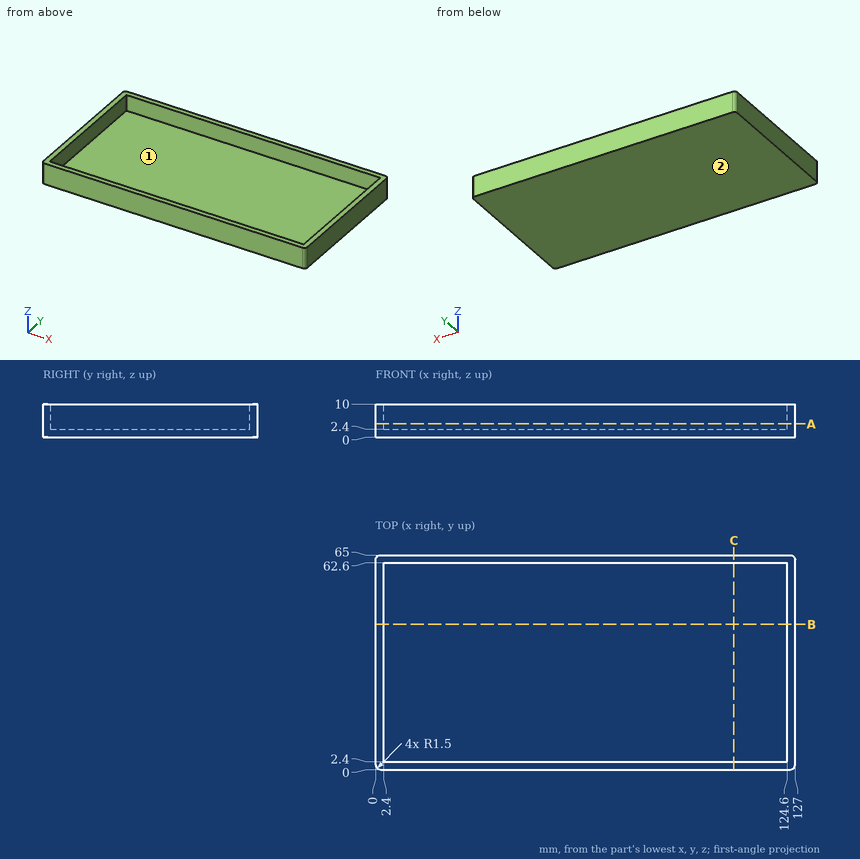
Part print with two shaded views. Sizes in mm from the minimum x, y, z corner. Give positions to 0.01 mm unless a question says otherwise; leave off trailing zeros. Write each loop counter-clockwise with the first axis right and the second up, starting at its lowest first coordinate (ties: lowest second). Pieces come first, ordered by that corner, then holes.
1) Cut at A-A on z = 4. Write the cut outline in (x, y).
Resolved:
outline: (0, 1.5) arc R1.5 ccw to (1.5, 0) - (125.5, 0) arc R1.5 ccw to (127, 1.5) - (127, 63.5) arc R1.5 ccw to (125.5, 65) - (1.5, 65) arc R1.5 ccw to (0, 63.5) - close; hole (2.4, 2.4) - (124.6, 2.4) - (124.6, 62.6) - (2.4, 62.6) - close
2) Cut at B-B on y = 44. Write the cut outline in (x, z), then the cut area to 3 significant figures.
Resolved:
outline: (0, 0) - (127, 0) - (127, 10) - (124.6, 10) - (124.6, 2.4) - (2.4, 2.4) - (2.4, 10) - (0, 10) - close
area: 341 mm2
3) Cut at C-C on x = 108.5. Write the cut outline in (y, z), then the cut area to 3 significant figures.
Resolved:
outline: (0, 0) - (65, 0) - (65, 10) - (62.6, 10) - (62.6, 2.4) - (2.4, 2.4) - (2.4, 10) - (0, 10) - close
area: 192 mm2
4) Probe L1, parallel to Y at x = 42, z = 5.75; L2, parallel to X at y = 48, z = 7.25; L3, parallel to Z at x = 66.5, y = 5. List the from-to ranges inside material, lowest first.
Resolved:
L1: y = 0 to 2.4, 62.6 to 65
L2: x = 0 to 2.4, 124.6 to 127
L3: z = 0 to 2.4
5) Pin check, flat tip, straight feed: pin 1 (2 mm diameter, centred on x = 107, y = 43.5, fed in from +Z). Stop position of the tip, or through.
Resolved:
pin 1: stops at z = 2.4
6) Two-plate mould, pull along X, no slides. Class the marked faces 1 and 2: released by +X, released by -X, zero draft, split by the parting line, or undercut.
Resolved:
face 1: undercut
face 2: zero draft
